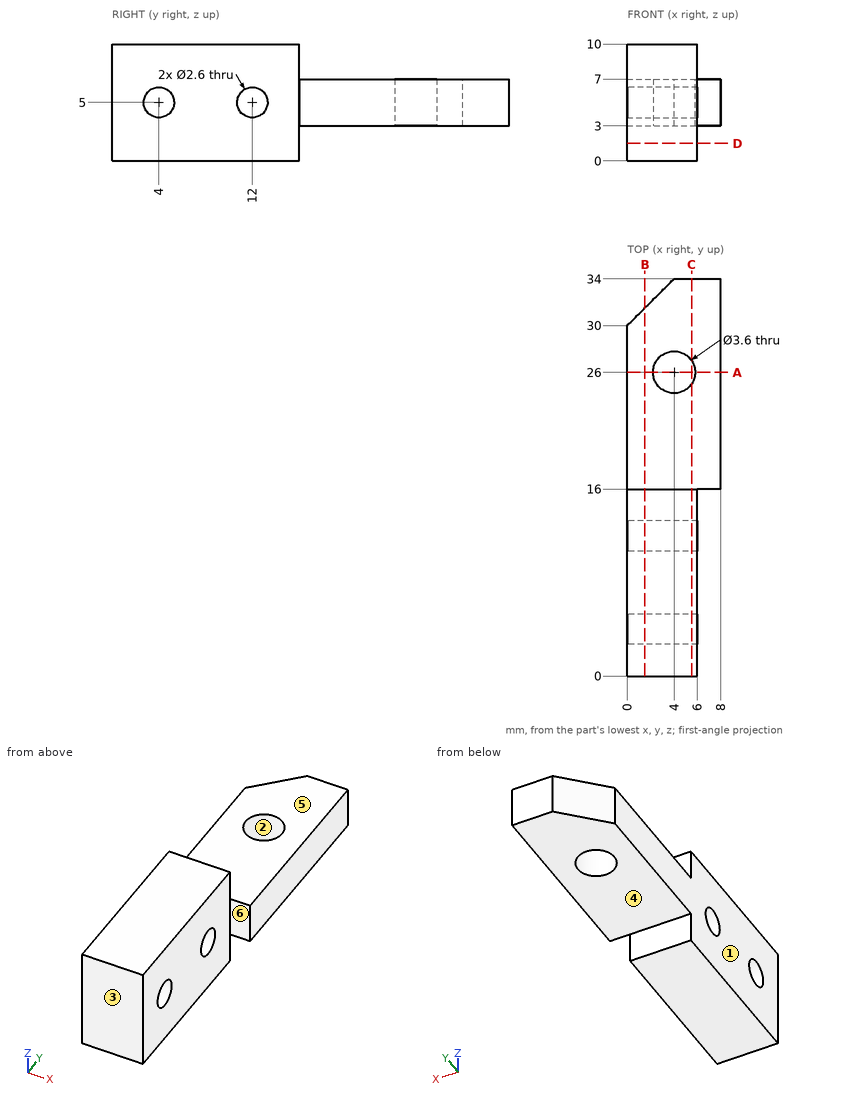
Here's the drawing with two shaded views (mm, measured from the low corner). I have some questions. A direction names the side the tool comes from. Coordinates: 2 decimals unless noted, no trailing zeros. Order: outer loops, then holes, each group sorted by start corner. A loop starts at its lowest first (then second) coordinate and runs counter-clockwise, first axis right, second up. Notation, with made-up numbers: (-21.75, -18.75) - (17.25, -18.75) arc R28 ccw to (17.25, 12.25) - close; hole circle Ø2 at (14.25, 83). An arc over 180 degrees is marked (long way). Answer in a Markdown table with one row per item. Add a question column.
(1) If we mould it in two halves opening along Y, with no side actions, what happens to the marked faces 1, 2 and 3? For each: released by +Y, released by -Y, zero draft, split by the parting line, or undercut.
(2) If we section it at C-C, the plane x = 5.5: Please give me the cut outline in (y, z), then the cut area to 3 significant figures.
(3) If we section it at B-B, the plane x = 1.5: Please give me the cut outline in (y, z), then the cut area to 3 significant figures.
(4) On a 3-axis mill with a long thin cutter (end or side, diameter ignored), from which of +Z, -Z, +X, -X, +Y, -Y can I reach the whole of each face in a straight line? I mean the marked faces 4, 5 and 6. Say none if no direction works.
(5) Will these pins go through, and if not, where does the flat tip stop? pin 1 (4 mm diameter, centred on x = 3.5, y = 25.5, fed in from +Z); pin 2 (3 mm diameter, centred on x = 4, y = 26, fed in from +Z); pin 3 (2.5 mm diameter, centred on x = 3, z = 1, fed in from +Y); pin 4 (5 mm diameter, centred on y = 7.5, z = 7, fed in from +X).
(6) If we section it at A-A, the plane y = 26: Please give me the cut outline in (x, z), then the cut area to 3 significant figures.
(7) If we section it at D-D, the plane z = 1.5: Please give me the cut outline in (x, y), then the cut area to 3 significant figures.
(8) I need wall thicknesses on L1, parallel to Y at x = 3.5, z = 5.5; L2, parallel to Z at x = 2.45, y = 4; L3, parallel to Y at x = 4, z = 8.75. Which ranges of each line are inside material? Lowest first, please.
Results are:
| question | item | result |
|---|---|---|
| 1 | face 1 | zero draft |
| 1 | face 2 | undercut |
| 1 | face 3 | released by -Y |
| 2 | outline | (0, 0) - (16, 0) - (16, 3) - (25.01, 3) - (25.01, 7) - (16, 7) - (16, 10) - (0, 10) - close; (26.99, 3) - (34, 3) - (34, 7) - (26.99, 7) - close; hole circle Ø2.6 at (4, 5); hole circle Ø2.6 at (12, 5) |
| 2 | area | 213 mm2 |
| 3 | outline | (0, 0) - (16, 0) - (16, 3) - (31.5, 3) - (31.5, 7) - (16, 7) - (16, 10) - (0, 10) - close; hole circle Ø2.6 at (4, 5); hole circle Ø2.6 at (12, 5) |
| 3 | area | 211 mm2 |
| 4 | face 4 | -Z, +X, -X, +Y |
| 4 | face 5 | +Z, +X, -X, +Y |
| 4 | face 6 | +Z, -Z, +X, -Y |
| 5 | pin 1 | stops at z = 7 |
| 5 | pin 2 | passes through |
| 5 | pin 3 | stops at y = 16 |
| 5 | pin 4 | stops at x = 6 |
| 6 | outline | (0, 3) - (2.2, 3) - (2.2, 7) - (0, 7) - close; (5.8, 3) - (8, 3) - (8, 7) - (5.8, 7) - close |
| 6 | area | 17.6 mm2 |
| 7 | outline | (0, 0) - (6, 0) - (6, 16) - (0, 16) - close |
| 7 | area | 96.0 mm2 |
| 8 | L1 | y = 0 to 2.8, 5.2 to 10.8, 13.2 to 24.27, 27.73 to 33.5 |
| 8 | L2 | z = 0 to 3.7, 6.3 to 10 |
| 8 | L3 | y = 0 to 16 |
